from build123d import *

# Parameters (mm, degrees)
SKETCH1_W           = 50.8
SKETCH1_H           = 38.1
SKETCH1_R           = 2.2479
BOSS_EXTRUDE1_DEPTH = 2.54
SKETCH4_W           = 50.8
SKETCH4_H           = 38.1
SKETCH4_R           = 5.08
SKETCH4_R_2         = 1.7018
BOSS_EXTRUDE2_DEPTH = 2.54
SKETCH5_R           = 2.2479
BOSS_EXTRUDE3_DEPTH = 2.54
BOSS_EXTRUDE4_START = 2.54
SKETCH6_R           = 2.25933
SKETCH6_R_2         = 2.2479
BOSS_EXTRUDE4_DEPTH = 2.54


with BuildPart() as part:
    # Sketch1 → Boss-Extrude1 (new body)
    with BuildSketch(Plane(origin=(0, 0, 0), x_dir=(1, 0, 0), z_dir=(0, 1, 0))):
        with Locations((25.4, 19.05)):
            Rectangle(SKETCH1_W, SKETCH1_H)
        with Locations(Location((6.35, 25.4, 0), (0, 0, 270))):
            Circle(SKETCH1_R, mode=Mode.SUBTRACT)
        with Locations(Location((19.05, 25.4, 0), (0, 0, 270))):
            Circle(SKETCH1_R, mode=Mode.SUBTRACT)
        with Locations(Location((31.75, 25.4, 0), (0, 0, 270))):
            Circle(SKETCH1_R, mode=Mode.SUBTRACT)
        with Locations(Location((44.45, 25.4, 0), (0, 0, 270))):
            Circle(SKETCH1_R, mode=Mode.SUBTRACT)
    extrude(amount=-BOSS_EXTRUDE1_DEPTH)

    # Sketch4 → Boss-Extrude2 (add)
    with BuildSketch(Plane.XY):
        with Locations((25.4, 16.51)):
            Rectangle(SKETCH4_W, SKETCH4_H)
        with Locations((25.4, 25.4)):
            Circle(SKETCH4_R, mode=Mode.SUBTRACT)
        with Locations((4.37642, 25.4)):
            Circle(SKETCH4_R_2, mode=Mode.SUBTRACT)
        with Locations((46.42358, 25.4)):
            Circle(SKETCH4_R_2, mode=Mode.SUBTRACT)
    extrude(amount=BOSS_EXTRUDE2_DEPTH)

    # Sketch5 → Boss-Extrude3 (add)
    with BuildSketch(Plane(origin=(50.8, 0, 0), x_dir=(0, 0, -1), z_dir=(1, 0, 0))):
        Polygon((0, 35.56), (-2.54, 35.56), (-2.54, -2.54), (38.1, -2.54), (38.1, 0), align=None)
        with Locations((11.803529412, 8.665882353)):
            Circle(SKETCH5_R, mode=Mode.SUBTRACT)
        with Locations((5.827058824, 19.871764706)):
            Circle(SKETCH5_R, mode=Mode.SUBTRACT)
    extrude(amount=BOSS_EXTRUDE3_DEPTH)

    # Sketch6 → Boss-Extrude4 (add)
    with BuildSketch(Plane.ZY.offset(BOSS_EXTRUDE4_START)):
        Polygon((0, 35.56), (-38.1, 0), (-38.1, -2.54), (2.54, -2.54), (2.54, 35.56), align=None)
        with Locations((-11.803529412, 8.665882353)):
            Circle(SKETCH6_R, mode=Mode.SUBTRACT)
        with Locations(Location((-5.827058824, 19.871764706, 0), (0, 0, 180))):
            Circle(SKETCH6_R_2, mode=Mode.SUBTRACT)
    extrude(amount=-BOSS_EXTRUDE4_DEPTH)


solid = part.part
CAD build for the part. Positions are in the model's coordinates, mm. A direction names the side the tool comes from. Coordinates: 2 decimals unless noted, no trailing zeros. Order: outer loops, then holes, each group sorted by start corner. A loop starts at its lowest first (then second) coordinate and runs counter-clockwise, first axis right, second up.
Item 1: Pin check, flat tip, straight feed: pin 1 Ø2 at (x, z) = (35, -16.5) entering from +Y. Stop position of the tip, or through.
Check sheet entries:
pin 1: stops at y = 0
Item 2: Drill centre lines: L1, parallel to X at y = -1.2, z = -25.4; L2, parallel to Y at x = 25.4, z = 0.8; L3, parallel to Y at x = 28, z = -23. Where is each one in solid material? Low to high.
Check sheet entries:
L1: x = -2.54 to 4.1, 8.6 to 16.8, 21.3 to 29.5, 34 to 42.2, 46.7 to 53.34
L2: y = -2.54 to 20.32, 30.48 to 35.56
L3: y = -2.54 to 0
Item 3: 3-axis set-ups, long thin cutter, end or side, ignore diameter. For faces 1 (the face through (45.969, -1.252, -27.057)), 2 (the face through (50.8, 10, -15)): which of +Z, -Z, +X, -X, +Y, -Y reach the whole face in a straight line?
Check sheet entries:
face 1: +Y, -Y
face 2: -Z, +Y
Item 4: Band-saw the part on A-A on x = 19.05. List the corners of the cut face in (y, z).
Check sheet entries:
outline: (-2.54, -38.1) - (0, -38.1) - (0, -27.65) - (-2.54, -27.65) - close; (-2.54, -23.15) - (0, -23.15) - (0, 0) - (35.56, 0) - (35.56, 2.54) - (-2.54, 2.54) - close
Item 5: Two-plate mould, pull along Y, no slides. Class faces 3 (the face through (4.155, 27.087, 1.252)), 4 (the face through (25, 18, 0)), 5 (the face through (-1.29, 6.46, -12.29)), 6 (the face through (52.05, 17.53, -19.32)): +Y half, -Y half, draft (parallel to the pull), parting line (faces both ways), or undercut.
Check sheet entries:
face 3: undercut
face 4: draft
face 5: undercut
face 6: +Y half
Item 6: Band-saw the part on B-B on y = 7.5. List the corners of the cut face in (x, z).
Check sheet entries:
outline: (-2.54, -30.06) - (0, -30.06) - (0, -13.74) - (-2.54, -13.74) - close; (-2.54, -9.87) - (0, -9.87) - (0, 0) - (50.8, 0) - (50.8, -9.88) - (53.34, -9.88) - (53.34, 2.54) - (-2.54, 2.54) - close; (50.8, -30.06) - (53.34, -30.06) - (53.34, -13.73) - (50.8, -13.73) - close
Item 7: Band-saw the part on C-C on z = -25. List the corners of the cut face in (x, y), plus the area to 3 significant figures.
Check sheet entries:
outline: (-2.54, -2.54) - (4.14, -2.54) - (4.14, 0) - (0, 0) - (0, 12.23) - (-2.54, 12.23) - close; (8.56, -2.54) - (16.84, -2.54) - (16.84, 0) - (8.56, 0) - close; (21.26, -2.54) - (29.54, -2.54) - (29.54, 0) - (21.26, 0) - close; (33.96, -2.54) - (42.24, -2.54) - (42.24, 0) - (33.96, 0) - close; (46.66, -2.54) - (53.34, -2.54) - (53.34, 12.23) - (50.8, 12.23) - (50.8, 0) - (46.66, 0) - close
area: 159 mm2
Item 8: Band-saw the part on D-D on y = 25.4. List the corners of the cut face in (x, z).
Check sheet entries:
outline: (-2.54, -10.89) - (0, -10.89) - (0, 0) - (2.67, 0) - (2.67, 2.54) - (-2.54, 2.54) - close; (6.08, 0) - (20.32, 0) - (20.32, 2.54) - (6.08, 2.54) - close; (30.48, 0) - (44.72, 0) - (44.72, 2.54) - (30.48, 2.54) - close; (48.13, 0) - (50.8, 0) - (50.8, -10.89) - (53.34, -10.89) - (53.34, 2.54) - (48.13, 2.54) - close
